For this review, use the dimensioned drawing (mm, ordinates from the lowest corner) and the shaded views. Coordinates: 2 decimals unless noted, no trailing zeros. Loops run counter-clockwise (first coordinate to the right, second up) from the corner with the lowest first, then second, coordinate; pieces in that order, holes last. Notation, with made-up numbers: (81.25, -27.75) - (111.25, -27.75) arc R20 ccw to (111.25, -4.75) - close; hole circle Ø9 at (35.5, 31.5). An arc over 180 degrees is marked (long way). Answer in a Markdown table with one row per item. Add a question column.
(1) We need section B-B, the plane x = 38. Write out the cut boundary in (y, z), plus the area to 3 significant figures.
(2) Clearance check with flat-ended pins moving along their axes: pin 1 (4 mm diameter, centred on x = 62, z = 87, fed in from -Y); pin 2 (12 mm diameter, centred on x = 44.5, z = 94.5, fed in from -Y); pin 3 (3 mm diameter, centred on x = 62, z = 4, fed in from -Y). State where each tip first meets the part, or that it passes through.
(3) The part is to be moulded in two halves that separate along X. For the marked faces 1 and 2, say which applies: released by +X, released by -X, zero draft, split by the parting line, or undercut.
(4) We need section A-A, the plane z = 87. Write out the cut boundary in (x, y).
(5) We need section D-D, the plane x = 62. Write out the cut boundary in (y, z).
(6) To check wall thickness, follow L1, parallel to X at y = 2.8, z = 4; L2, parallel to Z at x = 62, y = 4.1; L3, parallel to Z at x = 38, y = 2.75. State the ranges of each line that lie inside material, in increasing order. Write a range as [from, to].
(7) We need section C-C, the plane y = 4.5. Write out the cut boundary in (x, z), plus the area to 3 significant figures.
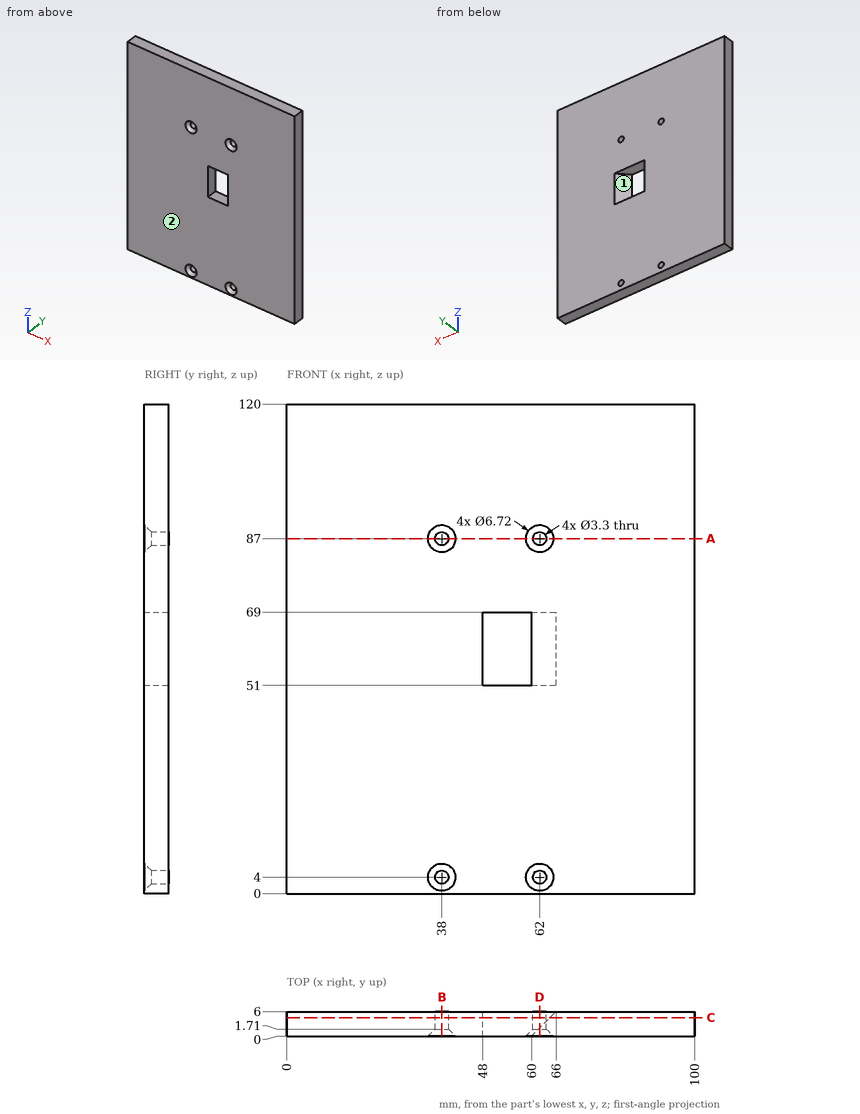
Responses:
| question | item | result |
|---|---|---|
| 1 | outline | (0, 0) - (6, 0) - (6, 2.35) - (1.71, 2.35) - (0, 0.64) - close; (0, 7.36) - (1.71, 5.65) - (6, 5.65) - (6, 85.35) - (1.71, 85.35) - (0, 83.64) - close; (0, 90.36) - (1.71, 88.65) - (6, 88.65) - (6, 120) - (0, 120) - close |
| 1 | area | 675 mm2 |
| 2 | pin 1 | stops at y = 1.36 |
| 2 | pin 2 | stops at y = 0 |
| 2 | pin 3 | passes through |
| 3 | face 1 | undercut |
| 3 | face 2 | zero draft |
| 4 | outline | (0, 0) - (34.64, 0) - (36.35, 1.71) - (36.35, 6) - (0, 6) - close; (39.65, 1.71) - (41.36, 0) - (58.64, 0) - (60.35, 1.71) - (60.35, 6) - (39.65, 6) - close; (63.65, 1.71) - (65.36, 0) - (100, 0) - (100, 6) - (63.65, 6) - close |
| 5 | outline | (0, 0) - (6, 0) - (6, 2.35) - (1.71, 2.35) - (0, 0.64) - close; (0, 7.36) - (1.71, 5.65) - (6, 5.65) - (6, 51) - (2, 51) - (2, 69) - (6, 69) - (6, 85.35) - (1.71, 85.35) - (0, 83.64) - close; (0, 90.36) - (1.71, 88.65) - (6, 88.65) - (6, 120) - (0, 120) - close |
| 6 | L1 | x = [0, 36.35], [39.65, 60.35], [63.65, 100] |
| 6 | L2 | z = [0, 2.35], [5.65, 51], [69, 85.35], [88.65, 120] |
| 6 | L3 | z = [0, 2.35], [5.65, 85.35], [88.65, 120] |
| 7 | outline | (0, 0) - (100, 0) - (100, 120) - (0, 120) - close; hole circle Ø3.3 at (38, 4); hole circle Ø3.3 at (38, 87); hole (48, 51) - (64.5, 51) - (64.5, 69) - (48, 69) - close; hole circle Ø3.3 at (62, 4); hole circle Ø3.3 at (62, 87) |
| 7 | area | 11,700 mm2 |
